Geometry: final body of the model. Coordinates: model frame, mm. A direction names the side the tool comes from. Give positions to 0.01 mm unless a question says otherwise; leave off trailing zeros. Order: outer loops, then holes, each group sorted by start corner. A loop starts at its lowest first (then second) coordinate and runs counter-clockwise, first axis right, second up. Notation, with made-up numbers: (36.5, -40) -> (75.5, -40) arc R28 cw to (75.5, -11) -> close; hole circle Ø7 at (36, 24). An arc over 180 degrees is marked (long way). Answer in a Markdown table with one row per item. Add a question column.
Q1. Line query: line 1 along Z through (x, y) = (0, 1.85); line 2 along X through (y, z) = (2.8, 48.5); line 3 along X through (y, z) = (0.75, -15.5). Output: solid intervals per line, ascending. Write a range as from..to.
Q2. Pull-direction query (X, two-part tool) for faces 3 (the face through (56.9, 1.48, 19.05)), 4 (the face through (-26.441, 1.479, -42.593)), 5 (the face through (-57.23, 1.48, 18.03)), 6 (the face through (-27, 1.48, -27.21)); classes: +X half, -X half, draft (parallel to the pull), parting line (faces both ways), or undercut.
Q3. Cut plane C-C on y = 1.15. Count the separate pieces of the cut face and the enclosed holes in it, and give its area (3 significant figures).
Q4. Cut plane B-B on z = -34. Return the cut outline in (x, y).
Q5. Cut plane A-A on z = -60. Return the cut outline in (x, y).
Q6. Contact query for a flat-ended pin moving along its axis: P1, Ø1, axis at x = 42, y = 1.5, coming from the -Z side. Output: stop coordinate, or through.
Q7. Set-up query: faces 1 (the face through (-17.731, 1.479, -34.357)), 2 (the face through (41.819, 1.479, 57.656)). Return all of +Z, -Z, +X, -X, +Y, -Y with unobstructed straight access to the full face (end or side cutting, diameter ignored); none if empty.
from build123d import *

# Parameters (mm, degrees)
ESQUISSE2_R        = 3.5
ESQUISSE2_R_2      = 1
BOSS_EXTRU_1_DEPTH = 3
CHANFREIN2_SIZE    = 5


with BuildPart() as part:
    # Esquisse2 → Boss.-Extru.1 (new body)
    with BuildSketch(Plane(origin=(0, 0, 0), x_dir=(1, 0, 0), z_dir=(0, 1, 0))):
        Polygon((70.534230275, 22.917960675), (0, 74.16407865), (-70.534230275, 22.917960675), (-43.59255168, -60), (43.59255168, -60), align=None)
        with Locations((-57.063390978, 18.541019662)):
            Circle(ESQUISSE2_R, mode=Mode.SUBTRACT)
        with Locations((0, 60)):
            Circle(ESQUISSE2_R, mode=Mode.SUBTRACT)
        with Locations((57.063390978, 18.541019662)):
            Circle(ESQUISSE2_R, mode=Mode.SUBTRACT)
        with Locations((35.267115138, -48.541019662)):
            Circle(ESQUISSE2_R, mode=Mode.SUBTRACT)
        with Locations((-35.267115138, -48.541019662)):
            Circle(ESQUISSE2_R, mode=Mode.SUBTRACT)
        with Locations((-62.769730075, 20.395121629)):
            Circle(ESQUISSE2_R_2, mode=Mode.SUBTRACT)
        with Locations((-51.35705188, 16.686917696)):
            Circle(ESQUISSE2_R_2, mode=Mode.SUBTRACT)
        with Locations((0, 66)):
            Circle(ESQUISSE2_R_2, mode=Mode.SUBTRACT)
        with Locations((0, 54)):
            Circle(ESQUISSE2_R_2, mode=Mode.SUBTRACT)
        with Locations((62.769730075, 20.395121629)):
            Circle(ESQUISSE2_R_2, mode=Mode.SUBTRACT)
        with Locations((51.35705188, 16.686917696)):
            Circle(ESQUISSE2_R_2, mode=Mode.SUBTRACT)
        with Locations((38.793826651, -53.395121629)):
            Circle(ESQUISSE2_R_2, mode=Mode.SUBTRACT)
        with Locations((31.740403624, -43.686917696)):
            Circle(ESQUISSE2_R_2, mode=Mode.SUBTRACT)
        with Locations((-38.793826651, -53.395121629)):
            Circle(ESQUISSE2_R_2, mode=Mode.SUBTRACT)
        with Locations((-31.740403624, -43.686917696)):
            Circle(ESQUISSE2_R_2, mode=Mode.SUBTRACT)
        with Locations((-3, -51.9)):
            Circle(ESQUISSE2_R_2, mode=Mode.SUBTRACT)
        with Locations((3, -51.9)):
            Circle(ESQUISSE2_R_2, mode=Mode.SUBTRACT)
        with Locations((3, -24.2)):
            Circle(ESQUISSE2_R_2, mode=Mode.SUBTRACT)
        with Locations((-3, -24.2)):
            Circle(ESQUISSE2_R_2, mode=Mode.SUBTRACT)
        with Locations((-23.942618677, -4.625041715)):
            Circle(ESQUISSE2_R_2, mode=Mode.SUBTRACT)
        with Locations((-22.088516711, -10.331380813)):
            Circle(ESQUISSE2_R_2, mode=Mode.SUBTRACT)
        with Locations((-48.432782213, -18.891151557)):
            Circle(ESQUISSE2_R_2, mode=Mode.SUBTRACT)
        with Locations((-50.286884179, -13.184812459)):
            Circle(ESQUISSE2_R_2, mode=Mode.SUBTRACT)
        with Locations((-11.797352122, 21.341567021)):
            Circle(ESQUISSE2_R_2, mode=Mode.SUBTRACT)
        with Locations((-16.651454089, 17.814855507)):
            Circle(ESQUISSE2_R_2, mode=Mode.SUBTRACT)
        with Locations((-32.933105577, 40.224626251)):
            Circle(ESQUISSE2_R_2, mode=Mode.SUBTRACT)
        with Locations((-28.079003611, 43.751337765)):
            Circle(ESQUISSE2_R_2, mode=Mode.SUBTRACT)
        with Locations((16.651454089, 17.814855507)):
            Circle(ESQUISSE2_R_2, mode=Mode.SUBTRACT)
        with Locations((11.797352122, 21.341567021)):
            Circle(ESQUISSE2_R_2, mode=Mode.SUBTRACT)
        with Locations((28.079003611, 43.751337765)):
            Circle(ESQUISSE2_R_2, mode=Mode.SUBTRACT)
        with Locations((32.933105577, 40.224626251)):
            Circle(ESQUISSE2_R_2, mode=Mode.SUBTRACT)
        with Locations((22.088516711, -10.331380813)):
            Circle(ESQUISSE2_R_2, mode=Mode.SUBTRACT)
        with Locations((23.942618677, -4.625041715)):
            Circle(ESQUISSE2_R_2, mode=Mode.SUBTRACT)
        with Locations((50.286884179, -13.184812459)):
            Circle(ESQUISSE2_R_2, mode=Mode.SUBTRACT)
        with Locations((48.432782213, -18.891151557)):
            Circle(ESQUISSE2_R_2, mode=Mode.SUBTRACT)
        Polygon((-5.85, -26.1), (5.85, -26.1), (5.85, -50), (1.5, -50), (1.5, -51.5), (-1.5, -51.5), (-1.5, -50), (-5.85, -50), align=None, mode=Mode.SUBTRACT)
        Polygon((-23.014825658, -13.629024174), (-45.745076398, -21.014530339), (-47.089300323, -16.877434493), (-48.515885098, -17.340959985), (-49.442936081, -14.487790436), (-48.016351306, -14.024264944), (-49.360575232, -9.887169098), (-26.630324492, -2.501662933), align=None, mode=Mode.SUBTRACT)
        Polygon((-20.073944502, 17.676799827), (-34.122012032, 37.012305993), (-30.602788106, 39.56917184), (-31.484465985, 40.782697332), (-29.057415001, 42.546053089), (-28.175737123, 41.332527597), (-24.656513198, 43.889393445), (-10.608445668, 24.553887279), align=None, mode=Mode.SUBTRACT)
        Polygon((10.608445668, 24.553887279), (24.656513198, 43.889393445), (28.175737123, 41.332527597), (29.057415001, 42.546053089), (31.484465985, 40.782697332), (30.602788106, 39.56917184), (34.122012032, 37.012305993), (20.073944502, 17.676799827), align=None, mode=Mode.SUBTRACT)
        Polygon((26.630324492, -2.501662933), (49.360575232, -9.887169098), (48.016351306, -14.024264944), (49.442936081, -14.487790436), (48.515885098, -17.340959985), (47.089300323, -16.877434493), (45.745076398, -21.014530339), (23.014825658, -13.629024174), align=None, mode=Mode.SUBTRACT)
    extrude(amount=BOSS_EXTRU_1_DEPTH)

    # Chanfrein2
    chanfrein2_edges = [part.edges().sort_by_distance(p)[0] for p in [
        (43.59255168, 1.5, 60),
        (-43.59255168, 1.5, 60),
        (-70.534230275, 1.5, -22.917960675),
        (0, 1.5, -74.16407865),
        (70.534230275, 1.5, -22.917960675),
    ]]
    chamfer(chanfrein2_edges, length=CHANFREIN2_SIZE)


solid = part.part
Completed:
| question | item | result |
|---|---|---|
| 1 | line 1 | z = -71.23..-67, -65..-63.5, -56.5..-55, -53..26.1, 51.5..60 |
| 1 | line 2 | x = -47.33..-38.77, -31.77..-5.85, 5.85..31.77, 38.77..47.33 |
| 1 | line 3 | x = -68.12..-58.8, -55.33..55.33, 58.8..68.12 |
| 2 | face 3 | +X half |
| 2 | face 4 | undercut |
| 2 | face 5 | -X half |
| 2 | face 6 | undercut |
| 3 | separate pieces | 1 |
| 3 | enclosed holes | 40 |
| 3 | area | 11,300 mm² |
| 4 | outline | (-55.28, 0) -> (-31.93, 0) -> (-31.93, 3) -> (-55.28, 3) -> close; (-17.47, 0) -> (17.47, 0) -> (17.47, 3) -> (-17.47, 3) -> close; (31.93, 0) -> (55.28, 0) -> (55.28, 3) -> (31.93, 3) -> close |
| 5 | outline | (-19.5, 0) -> (-3.5, 0) -> (-3.5, 3) -> (-19.5, 3) -> close; (3.5, 0) -> (19.5, 0) -> (19.5, 3) -> (3.5, 3) -> close |
| 6 | P1 | stops at z = -44.01 |
| 7 | face 1 | +Y, -Y |
| 7 | face 2 | +Z, +X, +Y, -Y |
